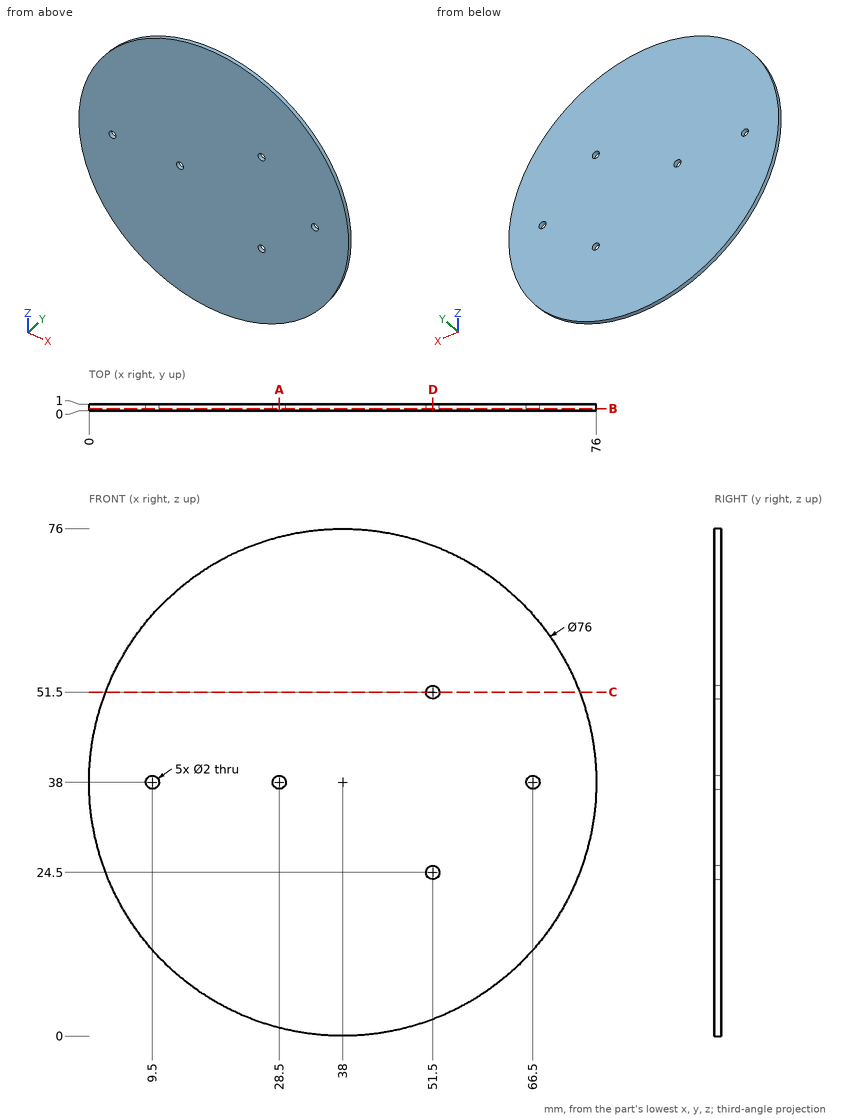
Here's the drawing with two shaded views (mm, measured from the low corner). I have some questions. Round coordinates to 2 decimals unless told otherwise and drop trailing zeros. Order: outer loops, then holes, each group sorted by start corner. A loop starts at its lowest first (then second) coordinate and runs counter-clockwise, first axis right, second up. Notation, with made-up numbers: M 43,23 L 91,23 A32 ccw 91,56 Z; hole C 27,10.5 d10. An arc over 180 degrees is marked long. Answer in a Markdown table with one row per item.
Item 1: Imagine slicing it at C-C, the plane z = 51.5. Write out the boundary of the cut face in (x, y).
A:
| item | result |
|---|---|
| outline | M 2.48,0 L 50.5,0 L 50.5,1 L 2.48,1 Z; M 52.5,0 L 73.52,0 L 73.52,1 L 52.5,1 Z |
Item 2: Imagine slicing it at D-D, the plane x = 51.5. Write out the boundary of the cut face in (y, z), and give its area (3 significant figures).
A:
| item | result |
|---|---|
| outline | M 0,2.48 L 1,2.48 L 1,23.5 L 0,23.5 Z; M 0,25.5 L 1,25.5 L 1,50.5 L 0,50.5 Z; M 0,52.5 L 1,52.5 L 1,73.52 L 0,73.52 Z |
| area | 67.0 mm2 |
Item 3: I'm going to push a flat-ended pin straight in: pin 1 (2.5 mm diameter, centred on x = 28.5, z = 38, fed in from -Y). Where does the tip first touch, or does it pass through?
A:
| item | result |
|---|---|
| pin 1 | stops at y = 0 |
Item 4: Imagine slicing it at A-A, the plane x = 28.5. Write out the boundary of the cut face in (y, z).
A:
| item | result |
|---|---|
| outline | M 0,1.21 L 1,1.21 L 1,37 L 0,37 Z; M 0,39 L 1,39 L 1,74.79 L 0,74.79 Z |
Item 5: If I drill on L1, parallel to X at y = 0.65, z = 38; L2, parallel to Z at x = 9.5, y = 0.3; L3, parallel to Z at x = 6, y = 0.75, over which ranges is the centre line in solid material (lowest first)? Write a range as from..to.
A:
| item | result |
|---|---|
| L1 | x = 0..8.5, 10.5..27.5, 29.5..65.5, 67.5..76 |
| L2 | z = 12.87..37, 39..63.13 |
| L3 | z = 17.51..58.49 |
Item 6: Imagine slicing it at B-B, the plane y = 0.3. Write out the boundary of the cut face in (x, z), and give its area (3 significant figures).
A:
| item | result |
|---|---|
| outline | C 38,38 d76; hole C 9.5,38 d2; hole C 28.5,38 d2; hole C 51.5,24.5 d2; hole C 51.5,51.5 d2; hole C 66.5,38 d2 |
| area | 4,520 mm2 |
